For this review, take the finished solid that the model builds, in its own axes (mm). Face numbers are marked on the shaded views. A direction names the side the tool comes from. Give positions to 0.01 mm unless a question says otherwise; leave off trailing zeros. Loops run counter-clockwise (first coordinate to the right, second up) from the corner with the lowest first, then second, coordinate; pieces in that order, holes last. Notation, with made-up numbers: (62, -10.75) - (90, -10.75) arc R23 ccw to (90, 14.25) - close; hole circle Ø5 at (70.25, 62). An arc over 180 degrees is marked (long way). Answer in a Markdown table with one row per item.
```python
from build123d import *

# Parameters (mm, degrees)
SKETCH1_W               = 34
SKETCH1_H               = 10
BOSS_EXTRUDE1_DEPTH     = 2
SKETCH2_W               = 2
SKETCH2_H               = 10
BOSS_EXTRUDE2_DEPTH     = 10
FILLET1_R               = 0.5
CUT_EXTRUDE1_DEPTH      = 37.400549446
CUT_EXTRUDE1_DEPTH_BACK = 37.400549446
SKETCH3_W               = 4
SKETCH3_H               = 6
CUT_EXTRUDE2_DEPTH      = 22.400934559
CUT_EXTRUDE2_DEPTH_BACK = 22.400934559


with BuildPart() as part:
    # Sketch1 → Boss-Extrude1 (new body)
    with BuildSketch(Plane.XY):
        Rectangle(SKETCH1_W, SKETCH1_H)
    extrude(amount=BOSS_EXTRUDE1_DEPTH)

    # Sketch2 → Boss-Extrude2 (add)
    with BuildSketch(Plane.XY.offset(2)):
        with Locations((-16, 0)):
            Rectangle(SKETCH2_W, SKETCH2_H)
        with Locations((16, 0)):
            Rectangle(SKETCH2_W, SKETCH2_H)
    extrude(amount=BOSS_EXTRUDE2_DEPTH)

    # Fillet1
    fillet1_edges = [part.edges().sort_by_distance(p)[0] for p in [
        (-15, 0, 2),
        (15, 0, 2),
    ]]
    fillet(fillet1_edges, radius=FILLET1_R)

    # Sketch3 → Cut-Extrude1 (cut, two sides: drawn at the far end of the back side and taken through both)
    with BuildSketch(Plane(origin=(17, 0, 0), x_dir=(0, 0, -1), z_dir=(1, 0, 0)).offset(-CUT_EXTRUDE1_DEPTH_BACK)):
        with Locations((-8, 0)):
            Rectangle(SKETCH3_W, SKETCH3_H)
    extrude(amount=CUT_EXTRUDE1_DEPTH + CUT_EXTRUDE1_DEPTH_BACK, mode=Mode.SUBTRACT)

    # Sketch4 → Cut-Extrude2 (cut, two sides: drawn at the far end of the back side and taken through both)
    with BuildSketch(Plane(origin=(0, 0, 0), x_dir=(-1, 0, 0), z_dir=(0, 0, -1)).offset(-CUT_EXTRUDE2_DEPTH_BACK)):
        with BuildLine():
            Line((-8, -1.5), (8, -1.5))
            ThreePointArc((8, -1.5), (9.5, 0), (8, 1.5))
            Line((8, 1.5), (-8, 1.5))
            ThreePointArc((-8, 1.5), (-9.5, 0), (-8, -1.5))
        make_face()
    extrude(amount=CUT_EXTRUDE2_DEPTH + CUT_EXTRUDE2_DEPTH_BACK, mode=Mode.SUBTRACT)


solid = part.part
```
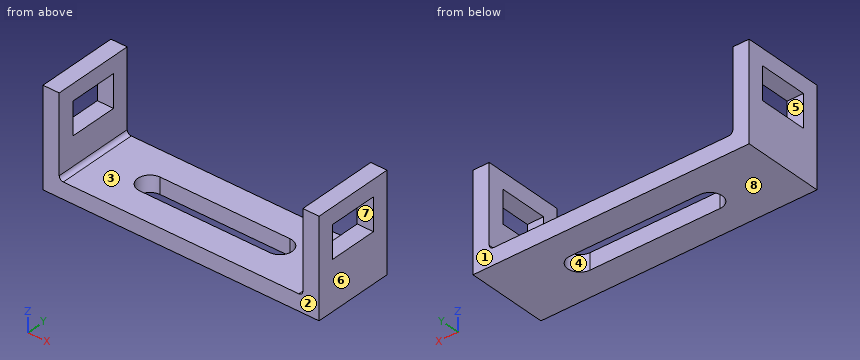
1. Wall thickness on line 1 (X direction, y = 1.25, z = 3); line 2 (Y direction, x = 15.5, z = 6.75); line 3 (Z direction, x = 9, y = -3.75): over which ranges is each line inside the solid? List them lowest first. Write a range as [from, to].
Values:
| item | result |
|---|---|
| line 1 | x = [-17, -15], [15, 17] |
| line 2 | y = [-5, -3], [3, 5] |
| line 3 | z = [0, 2] |
2. Clearance check with a flat-ended pin moving along its axis: pin 1 (4 mm diameter, centred on x = 10, y = 3, fed in from +Z). State where the tip first meets the part, or that it passes through.
Values:
| item | result |
|---|---|
| pin 1 | stops at z = 2 |
3. For the marked faces 1, 2, 3, 4 and 5, list the 3-axis set-ups (+Z, -Z, +X, -X, +Y, -Y) from which the entire face can be reached by the end or side of a thin tool; tool diameter is ignored.
Values:
| item | result |
|---|---|
| face 1 | +Z, -Z, +X, -X, +Y |
| face 2 | +Z, -Z, +X, -X, -Y |
| face 3 | +Z, +Y, -Y |
| face 4 | +Z, -Z |
| face 5 | +X, -X |
4. We need section B-B, the plane x = -5. Give the boundary of the cut face in (y, z).
Values:
| item | result |
|---|---|
| outline | (-5, 0) - (-1.5, 0) - (-1.5, 2) - (-5, 2) - close; (1.5, 0) - (5, 0) - (5, 2) - (1.5, 2) - close |
5. We need section C-C, the plane z = 9.5. Give the boundary of the cut face in (x, y).
Values:
| item | result |
|---|---|
| outline | (-17, -5) - (-15, -5) - (-15, -3) - (-17, -3) - close; (-17, 3) - (-15, 3) - (-15, 5) - (-17, 5) - close; (15, -5) - (17, -5) - (17, -3) - (15, -3) - close; (15, 3) - (17, 3) - (17, 5) - (15, 5) - close |
6. We need section D-D, the plane y = -2.25. Give the boundary of the cut face in (x, z).
Values:
| item | result |
|---|---|
| outline | (-17, 0) - (17, 0) - (17, 6) - (15, 6) - (15, 2.5) arc R0.5 cw to (14.5, 2) - (-14.5, 2) arc R0.5 cw to (-15, 2.5) - (-15, 6) - (-17, 6) - close; (-17, 10) - (-15, 10) - (-15, 12) - (-17, 12) - close; (15, 10) - (17, 10) - (17, 12) - (15, 12) - close |
7. Mouldability with a two-part tool opening along Z and no side actions: class the marked faces 6, 7 and 8 as released by +Z, released by -Z, zero draft, split by the parting line, or undercut.
Values:
| item | result |
|---|---|
| face 6 | zero draft |
| face 7 | undercut |
| face 8 | released by -Z |
8. We need section A-A, the plane z = 4. Give the boundary of the cut face in (x, y).
Values:
| item | result |
|---|---|
| outline | (-17, -5) - (-15, -5) - (-15, 5) - (-17, 5) - close; (15, -5) - (17, -5) - (17, 5) - (15, 5) - close |
